Part model, mm, in its own coordinate system. Face numbers are marked on the shaded views. A direction names the side the tool comes from. Coordinates: 2 decimals unless noted, no trailing zeros. Loops run counter-clockwise (first coordinate to the right, second up) from the corner with the lowest first, then second, coordinate; pieces in that order, holes last. Notation, with made-up numbers: M -20,17.5 L 13,17.5 A19 cw 13,54.5 Z; hole C -3.75,89.5 d5. An arc over 180 degrees is marked long. Use a Markdown table: item, result. Add a question column.
1) Wall check: probe 1 along Y at (x, z) = (-180.5, 53) (3 decimals); probe 2 along Z at (x, y) = (-164, -19) (3 decimals); probe 3 along Y at (x, z) = (-210.5, 67.5). Give the ranges that are in metal, low to high. Write a range as from..to.
2) Band-saw the part on A-A (z = 28). State how many separate pieces and enclosed holes the cut face has, plus the area to 3 significant figures.
3) Pull direction Y, two halves, no side cores. Call the marked faces 1, 2 and 3: released by +Y, released by -Y, zero draft, split by the parting line, or undercut.
4) Band-saw the part on D-D (z = 69.85). List the corners of the cut face in (x, y) (3 decimals), plus the area to 3 significant figures.
5) Pin check, flat tips, straight feed: pin 1 Ø2 at (y, z) = (-79, 63.5) entering from +X (3 decimals); pin 2 Ø12 at (x, y) = (-224.5, -107) entering from +Z (3 decimals); pin 3 Ø1 at (x, z) = (-171, 70.5) entering from +Y; pin 4 Ø1.5 at (x, z) = (-199.5, 86.5) entering from -Y. Stop position of each tip, or through.
6) Tool access for the marked faces 4 and 5: list every direction of +Z, -Z, +X, -X, +Y, -Y with a clear straight run to the whole face (end or side of a thin tool).
7) Band-saw the part on B-B (x = -101). List the corners of the cut face in (y, z) (3 decimals).
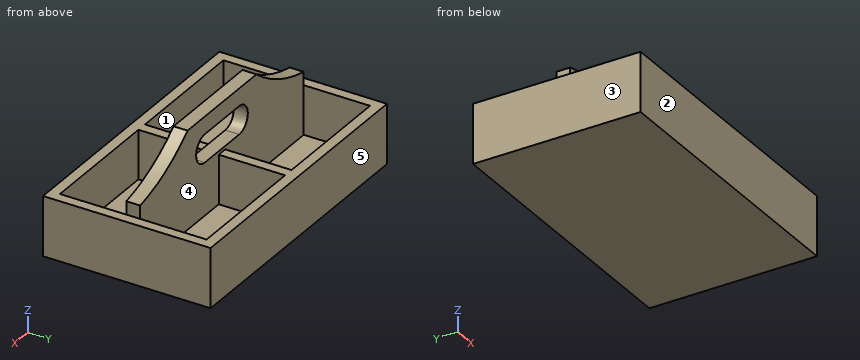
from build123d import *

# Parameters (mm, degrees)
F0_W      = 260.35
F0_H      = 9.525
F1_DEPTH  = 152.4
F3_DEPTH  = 44.45
F4_W      = 9.525
F4_H      = 133.35
F5_DEPTH  = 44.45
F7_DEPTH  = 44.45
F9_DEPTH  = 88.9
F11_DEPTH = 25.4
F12_DEPTH = 25.4
F14_DEPTH = 12.7
F15_W     = 9.525
F15_H     = 60.325
F16_DEPTH = 44.45


with BuildPart() as f1:
    # F0 (on Front) → F1 (new body)
    with BuildSketch(Plane.XZ):
        with Locations((-130.175, 4.7625)):
            Rectangle(F0_W, F0_H)
    extrude(amount=F1_DEPTH)

    # F2 (on face) → F3 (join)
    with BuildSketch(Plane.XY.offset(9.525)):
        Polygon((-260.35, 0), (-260.35, -9.525), (-248.4708428383, -9.525), (0, -9.525), (0, 0), align=None)
        Polygon((-260.35, -152.4), (-250.825, -152.4), (0, -152.4), (0, -142.875), (-260.35, -142.875), align=None)
    extrude(amount=F3_DEPTH)

    # F4 (on face) → F5 (join)
    with BuildSketch(Plane.XY.offset(9.525)):
        with Locations((-255.5875, -76.2)):
            Rectangle(F4_W, F4_H)
        with Locations((-4.7625, -76.2)):
            Rectangle(F4_W, F4_H)
    extrude(amount=F5_DEPTH)

    # F6 (on face) → F7 (join)
    with BuildSketch(Plane.XY.offset(9.525)):
        Polygon((-134.9375, -82.55), (-134.9375, -142.875), (-130.175, -142.875), (-125.4125, -142.875), (-125.4125, -82.55), align=None)
    extrude(amount=F7_DEPTH)

    # F8 (on face) → F9 (join)
    with BuildSketch(Plane.XY.offset(9.525)):
        Polygon((-250.825, -69.85), (-250.825, -82.55), (-134.9375, -82.55), (-125.4125, -82.55), (-9.525, -82.55), (-9.525, -69.85), align=None)
    extrude(amount=F9_DEPTH)

    # F10 (on face) → F11 (join)
    with BuildSketch(Plane.XZ.offset(82.55)):
        with BuildLine():
            Line((-180.975, 98.425), (-250.825, 98.425))
            Line((-250.825, 98.425), (-250.825, 65.953187989))
            ThreePointArc((-250.825, 65.953187989), (-213.8145902973, 77.7031765567), (-180.975, 98.425))
        make_face()
        with BuildLine():
            Line((-250.825, 65.953187989), (-250.825, 98.425))
            Line((-250.825, 98.425), (-180.975, 98.425))
            ThreePointArc((-180.975, 98.425), (-149.1074694289, 134.677129134), (-130.175, 179.0766558518))
            ThreePointArc((-130.175, 179.0766558518), (-134.6905811935, 215.9), (-130.175, 252.7233441482))
            ThreePointArc((-130.175, 252.7233441482), (-406.0727955672, 298.5942281561), (-250.825, 65.953187989))
        make_face()
        with BuildLine():
            ThreePointArc((-125.6594188065, 215.9), (-126.7925264835, 234.44958994), (-130.175, 252.7233441482))
            ThreePointArc((-130.175, 252.7233441482), (-134.6905811935, 215.9), (-130.175, 179.0766558518))
            ThreePointArc((-130.175, 179.0766558518), (-126.7925264835, 197.35041006), (-125.6594188065, 215.9))
        make_face()
        with BuildLine():
            ThreePointArc((170.1094188065, 215.9), (36.2590087465, 367.166892323), (-130.175, 252.7233441482))
            ThreePointArc((-130.175, 252.7233441482), (-126.7925264835, 234.44958994), (-125.6594188065, 215.9))
            ThreePointArc((-125.6594188065, 215.9), (-126.7925264835, 197.35041006), (-130.175, 179.0766558518))
            ThreePointArc((-130.175, 179.0766558518), (-111.2425305711, 134.677129134), (-79.375, 98.425))
            ThreePointArc((-79.375, 98.425), (82.632814335, 78.0206588605), (170.1094188065, 215.9))
        make_face()
    extrude(amount=-F11_DEPTH)

    # F10 (on face) → F12 (cut)
    with BuildSketch(Plane.XZ.offset(82.55)):
        with BuildLine():
            Line((-180.975, 98.425), (-250.825, 98.425))
            Line((-250.825, 98.425), (-250.825, 65.953187989))
            ThreePointArc((-250.825, 65.953187989), (-213.8145902973, 77.7031765567), (-180.975, 98.425))
        make_face()
        with BuildLine():
            Line((-250.825, 65.953187989), (-250.825, 98.425))
            Line((-250.825, 98.425), (-180.975, 98.425))
            ThreePointArc((-180.975, 98.425), (-149.1074694289, 134.677129134), (-130.175, 179.0766558518))
            ThreePointArc((-130.175, 179.0766558518), (-134.6905811935, 215.9), (-130.175, 252.7233441482))
            ThreePointArc((-130.175, 252.7233441482), (-406.0727955672, 298.5942281561), (-250.825, 65.953187989))
        make_face()
        with BuildLine():
            ThreePointArc((-125.6594188065, 215.9), (-126.7925264835, 234.44958994), (-130.175, 252.7233441482))
            ThreePointArc((-130.175, 252.7233441482), (-134.6905811935, 215.9), (-130.175, 179.0766558518))
            ThreePointArc((-130.175, 179.0766558518), (-126.7925264835, 197.35041006), (-125.6594188065, 215.9))
        make_face()
        with BuildLine():
            ThreePointArc((170.1094188065, 215.9), (36.2590087465, 367.166892323), (-130.175, 252.7233441482))
            ThreePointArc((-130.175, 252.7233441482), (-126.7925264835, 234.44958994), (-125.6594188065, 215.9))
            ThreePointArc((-125.6594188065, 215.9), (-126.7925264835, 197.35041006), (-130.175, 179.0766558518))
            ThreePointArc((-130.175, 179.0766558518), (-111.2425305711, 134.677129134), (-79.375, 98.425))
            ThreePointArc((-79.375, 98.425), (82.632814335, 78.0206588605), (170.1094188065, 215.9))
        make_face()
    extrude(amount=-F12_DEPTH, mode=Mode.SUBTRACT)

    # F13 (on face) → F14 (cut)
    with BuildSketch(Plane.XZ.offset(82.55)):
        with BuildLine():
            Line((-104.775, 82.55), (-155.575, 82.55))
            ThreePointArc((-155.575, 82.55), (-168.275, 69.85), (-155.575, 57.15))
            Line((-155.575, 57.15), (-104.775, 57.15))
            ThreePointArc((-104.775, 57.15), (-92.075, 69.85), (-104.775, 82.55))
        make_face()
    extrude(amount=-F14_DEPTH, mode=Mode.SUBTRACT)

    # F15 (on face) → F16 (join)
    with BuildSketch(Plane.XY.offset(9.525)):
        with Locations((-130.175, -39.6875)):
            Rectangle(F15_W, F15_H)
    extrude(amount=F16_DEPTH)


solid = f1.part
Entries:
| question | item | result |
|---|---|---|
| 1 | probe 1 | -152.4..-142.875, -82.55..-69.85, -9.525..0 |
| 1 | probe 2 | 0..9.525 |
| 1 | probe 3 | -82.55..-69.85 |
| 2 | separate pieces | 1 |
| 2 | enclosed holes | 4 |
| 2 | area | 11,700 mm2 |
| 3 | face 1 | undercut |
| 3 | face 2 | released by -Y |
| 3 | face 3 | zero draft |
| 4 | outline | M -234.526,-82.55 L -168.275,-82.55 L -168.275,-69.85 L -234.526,-69.85 Z; M -92.075,-82.55 L -25.824,-82.55 L -25.824,-69.85 L -92.075,-69.85 Z |
| 4 | area | 1,680 mm2 |
| 5 | pin 1 | x = -9.525 |
| 5 | pin 2 | z = 9.525 |
| 5 | pin 3 | y = -69.85 |
| 5 | pin 4 | through |
| 6 | face 4 | +Z |
| 6 | face 5 | +Z, -Z, +X, -X, +Y |
| 7 | outline | M -152.4,0 L 0,0 L 0,53.975 L -9.525,53.975 L -9.525,9.525 L -69.85,9.525 L -69.85,57.724 L -82.55,57.724 L -82.55,9.525 L -142.875,9.525 L -142.875,53.975 L -152.4,53.975 Z; M -82.55,81.976 L -69.85,81.976 L -69.85,98.425 L -82.55,98.425 Z |
